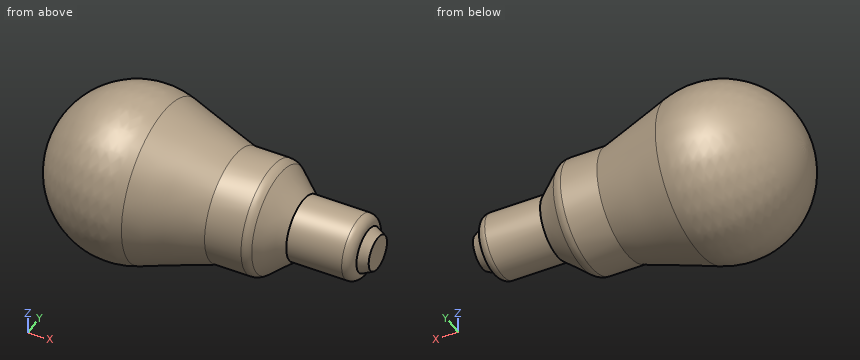
```python
from build123d import *


with BuildPart() as f1:
    # F0 (on Top) → F1 (revolve)
    with BuildSketch(Plane.XY):
        with BuildLine():
            Line((48.162115, 20), (35, 20))
            Line((35, 20), (9.442773, 28.475148))
            ThreePointArc((9.442773, 28.475148), (-17.560137, 24.323684), (-30, 0))
            Line((-30, 0), (87, 0))
            Line((87, 0), (87, 6.25))
            Line((87, 6.25), (83.5, 8))
            ThreePointArc((83.5, 8), (82.474874, 10.474874), (80, 11.5))
            Line((80, 11.5), (60, 11.5))
            Line((60, 11.5), (51.400357, 18.809697))
            ThreePointArc((51.400357, 18.809697), (49.887154, 19.692999), (48.162115, 20))
        make_face()
    revolve(axis=Axis((17.5, 0, 0), (1, 0, 0)))


solid = f1.part
```
For this review, take the finished solid that the model builds, in its own axes (mm). Give positions to 0.01 mm unless a question says otherwise; leave off trailing zeros. Order: outer loops, then holes, each group sorted by start corner. A loop starts at its lowest first (then second) coordinate and runs counter-clockwise, first axis right, second up.
1) Insertion check: pin 1 (1.5 mm diameter, centred on x = 14.5, z = 2.5, fed in from +Y); pin 2 (12 mm diameter, centred on x = 52, z = -3.5, fed in from +Y); pin 3 (12 mm diameter, centred on x = 50, y = 20.5, fed in from +Z). Each pin has a flat end and moves straight along its axis. Give the tip position at first contact, or say it passes through.
2) Wall thickness on line 1 (X direction, y = -8, z = 9); line 2 (Z direction, x = 3.5, y = 5.5); line 3 (X direction, y = 13, z = 16): over which ranges is each line inside the solid? List them lowest first.
3) Take a section at A-A (x = 26). Give the boundary of the cut face in (y, z).
Derived:
1. pin 1: stops at y = 26.94
1. pin 2: stops at y = 20
1. pin 3: stops at z = 13.59
2. line 1: x = -27.48 to 59.36
2. line 2: z = -29.28 to 29.28
2. line 3: x = -21.79 to 33.14
3. outline: circle Ø45.97 at (0, 0)
